Model file for the job. Use its own axes, mm. Give positions to 0.01 mm unless a question says otherwise; leave off trailing zeros. Order: outer loops, then holes, each group sorted by start corner. A loop starts at its lowest first (then second) coordinate and runs counter-clockwise, first axis right, second up. Notation, with made-up numbers: (35.5, 50) -> (39.5, 50) arc R14 cw to (39.5, 56) -> close; hole circle Ø10 at (84, -3). An arc over 180 degrees is marked (long way). Answer in a Markdown table with one row per item. Add a question column.
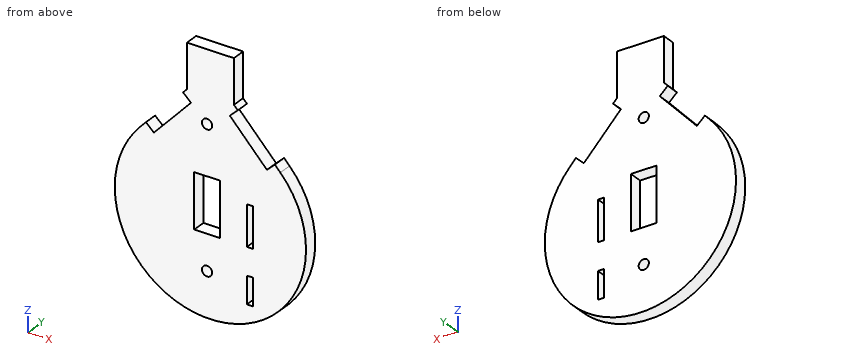
from build123d import *

# Parameters (mm, degrees)
F0_R     = 2.3876
F0_W     = 11.9644477963
F0_H     = 25.4
F0_W_2   = 2.794
F0_H_2   = 12.7
F0_H_3   = 18.8976
F1_DEPTH = 3.175
F3_W     = 6.35
F3_H     = 25.4
F4_DEPTH = 5.08
F6_W     = 6.35
F6_H     = 25.4
F7_DEPTH = 5.08


with BuildPart() as f1:
    # F0 (on Front) → F1 (new body, symmetric)
    with BuildSketch(Plane.XZ):
        with BuildLine():
            Line((-9.4017383467, 23.2221963037), (-31.0533456504, 0))
            ThreePointArc((-31.0533456504, 0), (1.5738401562, -75.0292582617), (34.2010259628, 0))
            Line((34.2010259628, 0), (12.5494186591, 23.2221963037))
            Line((12.5494186591, 23.2221963037), (12.5494186591, 43.8596963037))
            Line((12.5494186591, 43.8596963037), (-9.4017383467, 43.8596963037))
            Line((-9.4017383467, 43.8596963037), (-9.4017383467, 23.2221963037))
        make_face()
        with Locations((0, -54.2525947094)):
            Circle(F0_R, mode=Mode.SUBTRACT)
        with Locations((0, -25.0313151628)):
            Rectangle(F0_W, F0_H, mode=Mode.SUBTRACT)
        with Locations((19.9750838982, -56.7813151628)):
            Rectangle(F0_W_2, F0_H_2, mode=Mode.SUBTRACT)
        with Locations((19.9750838982, -28.2825151628)):
            Rectangle(F0_W_2, F0_H_3, mode=Mode.SUBTRACT)
        with Locations((0, 10.739565827)):
            Circle(F0_R, mode=Mode.SUBTRACT)
    extrude(amount=F1_DEPTH, both=True)

    # F3 (on offset) → F4 (cut)
    with BuildSketch(Plane(origin=(-16.6122141895, 0, 15.4886787354), x_dir=(0, -1, 0), z_dir=(-0.7314077576, 0, 0.6819403875))):
        with Locations((0, -4.733831039)):
            Rectangle(F3_W, F3_H)
    extrude(amount=-F4_DEPTH, mode=Mode.SUBTRACT)

    # F6 (on offset) → F7 (cut)
    with BuildSketch(Plane(origin=(18.2960887755, 0, 17.0586676721), x_dir=(0, 1, 0), z_dir=(0.7314077576, 0, 0.6819403875))):
        with Locations((0, -6.8803708986)):
            Rectangle(F6_W, F6_H)
    extrude(amount=-F7_DEPTH, mode=Mode.SUBTRACT)


solid = f1.part
Item 1: Saw through at D-D on y = 1.5. List the corners of the cut face in (x, z), plus the area to 3 significant figures.
Item 2: Pin check, flat tips, straight feed: pin 1 Ø0.8 at (x, y) = (20, -1) entering from +Z; pin 2 Ø3 at (y, z) = (-1, 29) entering from +X; pin 3 Ø1.9 at (x, y) = (2.5, 0) entering from -Z; pin 4 Ø3 at (y, z) = (-0.5, -29.5) entering from -X. Stop position of each tip, or through.
Item 3: Wall check: line 1 (X direction, y = -0.25, z = -25); line 2 (Z direction, x = 0, y = 0) (3 decimals); line 3 (X direction, y = -1.5, z = -27). Give the ranges that are in metal, low to high.
Item 4: Saw through at B-B on z = -21.5. List the corners of the cut face in (x, y) (3 decimals), plus the area to 3 significant figures.
Item 5: Saw through at C-C on z = -59. List the corners of the cut face in (x, y) (3 decimals).
Item 6: Saw through at A-A on x = 0. List the corners of the cut face in (y, z) (3 decimals).
Evaluation:
| question | item | result |
|---|---|---|
| 1 | outline | (-31.05, 0) arc R44.61 ccw (long way) to (34.2, 0) -> (31.65, 2.74) -> (27.93, -0.73) -> (10.61, 17.85) -> (14.33, 21.32) -> (12.55, 23.22) -> (12.55, 43.86) -> (-9.4, 43.86) -> (-9.4, 23.22) -> (-11.18, 21.32) -> (-7.46, 17.85) -> (-24.79, -0.73) -> (-28.5, 2.74) -> close; hole (-5.98, -37.73) -> (5.98, -37.73) -> (5.98, -12.33) -> (-5.98, -12.33) -> close; hole circle Ø4.78 at (0, -54.25); hole circle Ø4.78 at (0, 10.74); hole (18.58, -63.13) -> (21.37, -63.13) -> (21.37, -50.43) -> (18.58, -50.43) -> close; hole (18.58, -37.73) -> (21.37, -37.73) -> (21.37, -18.83) -> (18.58, -18.83) -> close |
| 1 | area | 6,390 mm2 |
| 2 | pin 1 | stops at z = 8.21 |
| 2 | pin 2 | stops at x = 12.55 |
| 2 | pin 3 | stops at z = -75.03 |
| 2 | pin 4 | stops at x = -43.03 |
| 3 | line 1 | x = -42.7 to -5.98, 5.98 to 18.58, 21.37 to 45.85 |
| 3 | line 2 | z = -75.001 to -56.64, -51.865 to -37.731, -12.331 to 8.352, 13.127 to 43.86 |
| 3 | line 3 | x = -42.9 to -5.98, 5.98 to 18.58, 21.37 to 46.05 |
| 4 | outline | (-42.134, -3.175) -> (-5.982, -3.175) -> (-5.982, 3.175) -> (-42.134, 3.175) -> close; (5.982, -3.175) -> (18.578, -3.175) -> (18.578, 3.175) -> (5.982, 3.175) -> close; (21.372, -3.175) -> (45.282, -3.175) -> (45.282, 3.175) -> (21.372, 3.175) -> close |
| 4 | area | 461 mm2 |
| 5 | outline | (-32.677, -3.175) -> (18.578, -3.175) -> (18.578, 3.175) -> (-32.677, 3.175) -> close; (21.372, -3.175) -> (35.825, -3.175) -> (35.825, 3.175) -> (21.372, 3.175) -> close |
| 6 | outline | (-3.175, -75.001) -> (3.175, -75.001) -> (3.175, -56.64) -> (-3.175, -56.64) -> close; (-3.175, -51.865) -> (3.175, -51.865) -> (3.175, -37.731) -> (-3.175, -37.731) -> close; (-3.175, -12.331) -> (3.175, -12.331) -> (3.175, 8.352) -> (-3.175, 8.352) -> close; (-3.175, 13.127) -> (3.175, 13.127) -> (3.175, 43.86) -> (-3.175, 43.86) -> close |
